```python
from build123d import *


with BuildPart() as part:
    # Sketch1 → Revolve1 (revolve)
    with BuildSketch(Plane(origin=(0, 0, 0), x_dir=(0, 0, -1), z_dir=(1, 0, 0)), mode=Mode.PRIVATE) as revolve1_sk:
        Polygon((-4.5, 7.3), (-4.5, 6.3), (-4.3, 6.1), (-4.5, 5.9), (-4.5, 4.41), (-4.3, 4.25), (-4.5, 4), (-4.5, 2.5), (0, 2.5), (0, 12), (-2.5, 12), (-4.5, 9.5), (-4.5, 7.7), (-4.3, 7.5), align=None)
    revolve(revolve1_sk.sketch.rotate(Axis((0, 0, 0), (0, 0, 1)), 90), axis=Axis((0, 0, 0), (0, 0, 1)))

    # Mirror1: part across plane


with BuildPart() as part_1:
    add(part.part)
    add(part.part.mirror(Plane(origin=(0, 2.5, 0), x_dir=(1, 0, 0), z_dir=(0, 0, -1))))


solid = part_1.part
```
Read the model definition and answer for the solid it produces. Units are mm, in the model's axes. Coordinates: 2 decimals unless noted, no trailing zeros. Write each loop counter-clockwise with the first axis right and the second up, starting at its lowest first coordinate (ties: lowest second). Pieces come first, ordered by that corner, then holes. Notation, with made-up numbers: (4.5, 78) -> (39.5, 78) arc R24 ccw to (39.5, 93) -> close; hole circle Ø8 at (-30, 61.5). An arc over 180 degrees is marked (long way). Write item = value, one per line.
(1) Section B-B on z = 3.25 is taken. Write down the section's boundary in (x, y) (1 decimal), plus the area to 3 significant figures.
From the geometry:
outline = circle Ø22.1 at (0, 0); hole circle Ø5 at (0, 0)
area = 365 mm2
(2) Given pin 1 Ø4 at (x, y) = (4.5, 9) entering from +Z; pin 2 Ø4 at (x, z) = (2.5, 2) entering from +Y; pin 3 Ø4 at (y, z) = (-4.5, 2) entering from +X, each flat-ended and moving along its own axis, determine where each tip first touches the part or whether it passes through.
From the geometry:
pin_1 = 4.5
pin_2 = 11.99
pin_3 = 11.74
(3) Straight lines are drawn through the part: L1, parallel to Y at x = 0, z = -1.05; L2, parallel to Y at x = 0, z = 2.65; L3, parallel to X at y = -1.25, z = -4. For each, find the intervals that lie inside material, in ascending order. Write a range as from..to.
From the geometry:
L1 = -12..-2.5, 2.5..12
L2 = -11.81..-2.5, 2.5..11.81
L3 = -10.05..-2.17, 2.17..10.05
(4) Section A-A on z = -3.75 is taken. Write down the section's boundary in (x, y) (1 decimal), plus the area to 3 significant figures.
From the geometry:
outline = circle Ø20.9 at (0, 0); hole circle Ø5 at (0, 0)
area = 323 mm2
